```python
from build123d import *

# Parameters (mm, degrees)
SKETCH1_W           = 7
SKETCH1_H           = 5
BOSS_EXTRUDE1_DEPTH = 31


with BuildPart() as part:
    # Sketch1 → Boss-Extrude1 (new body)
    with BuildSketch(Plane(origin=(0, 0, 0), x_dir=(1, 0, 0), z_dir=(0, 1, 0))):
        with Locations((0, 28.5)):
            Rectangle(SKETCH1_W, SKETCH1_H)
        with Locations((0, 33.5)):
            Rectangle(SKETCH1_W, SKETCH1_H)
        Polygon((-3.5, 31), (-17, 31), (-17, -31), (17, -31), (17, 31), (3.5, 31), (3.5, 26), (-3.5, 26), align=None)
    extrude(amount=BOSS_EXTRUDE1_DEPTH)


solid = part.part
```
The model under review builds one solid part; all positions refer to its coordinate system, in mm. A direction names the side the tool comes from. Give positions to 0.01 mm unless a question says otherwise; leave off trailing zeros. Write each loop counter-clockwise with the first axis right and the second up, starting at its lowest first coordinate (ties: lowest second). Pieces come first, ordered by that corner, then holes.
(1) Consider section A-A, the plane y = 16. Give the boundary of the cut face in (x, z), and give its area (3 significant figures).
(2) Tool access review of faces 1 (the flat face through (10, 15, -31)), 2 (the flat face through (-10, 15, -31)), 3 (the flat face through (0, 31, -3)): name each direction out of +Z, -Z, +X, -X, +Y, -Y from which nothing blocks a thin tool from reaching the whole face with its end or side.
(3) For P1, Ø12, axis at x = -7, z = 15, coming from the -Y side; P2, Ø8, axis at x = 10.5, y = 18, coming from the -Z side; P3, Ø5.5, axis at y = 19.5, z = -34.5, coming from the -X side, all flat-tipped, find the tip position at first contact; note any pin that passes through.
(4) To check wall thickness, follow L1, parallel to Z at x = 9, y = 13.5. State the ranges of the line that lie inside material, in increasing order.
(5) Consider section B-B, the plane x = -5. Give the boundary of the cut face in (y, z).
Returned:
1. outline: (-17, -31) - (-3.5, -31) - (-3.5, -36) - (3.5, -36) - (3.5, -31) - (17, -31) - (17, 31) - (-17, 31) - close
1. area: 2,140 mm2
2. face 1: -Z, +X, +Y, -Y
2. face 2: -Z, -X, +Y, -Y
2. face 3: +Z, -Z, +X, -X, +Y
3. P1: stops at y = 0
3. P2: stops at z = -31
3. P3: stops at x = -3.5
4. L1: z = -31 to 31
5. outline: (0, -31) - (31, -31) - (31, 31) - (0, 31) - close
